from build123d import *

# Parameters (mm, degrees)
F0_R     = 3
F1_DEPTH = 2
F2_DEPTH = 5
F3_DEPTH = 9
F4_R     = 2.5
F5_DEPTH = 4
F7_DEPTH = 1
F10_D    = 2


with BuildPart() as f1:
    # F0 (on Front) → F1 (new body)
    with BuildSketch(Plane.XZ):
        with BuildLine():
            ThreePointArc((-5.5, 0), (0, 5.5), (5.5, 0))
            Line((5.5, 0), (5.5, 30))
            ThreePointArc((5.5, 30), (0, 35.5), (-5.5, 30))
            Line((-5.5, 30), (-5.5, 0))
        make_face()
        with Locations((0, 30)):
            Circle(F0_R, mode=Mode.SUBTRACT)
    extrude(amount=F1_DEPTH)

    # F0 (on Front) → F2 (join)
    with BuildSketch(Plane.XZ):
        with BuildLine():
            ThreePointArc((-5.5, 0), (0, -5.5), (5.5, 0))
            ThreePointArc((5.5, 0), (0, 5.5), (-5.5, 0))
        make_face()
        Polygon((2.8867513459, 0), (1.443375673, -2.5), (-1.443375673, -2.5), (-2.8867513459, 0), (-1.443375673, 2.5), (1.443375673, 2.5), align=None, mode=Mode.SUBTRACT)
    extrude(amount=F2_DEPTH)

    # F0 (on Front) → F3 (join)
    with BuildSketch(Plane.XZ):
        Polygon((-1.443375673, -2.5), (1.443375673, -2.5), (2.8867513459, 0), (1.443375673, 2.5), (-1.443375673, 2.5), (-2.8867513459, 0), align=None)
    extrude(amount=F3_DEPTH)

    # F4 (on face) → F5 (cut)
    with BuildSketch(Plane.XZ):
        Circle(F4_R)
    extrude(amount=F5_DEPTH, mode=Mode.SUBTRACT)

    # F6 (on Right) → F7 (join, symmetric)
    with BuildSketch(Plane.YZ):
        Polygon((-5, 5.5), (-5, 3.9388309233), (0, 3.9388309233), (0, 23.931786418), (-1.7340160995, 24.0223151183), align=None)
    extrude(amount=F7_DEPTH, both=True)

    # F10 (through all)
    with Locations(Plane(origin=(4.7631397208, 0, -2.75), x_dir=(0, 1, 0), z_dir=(0.8660254038, 0, -0.5))):
        with Locations((-2, 0)):
            Hole(F10_D / 2)


solid = f1.part
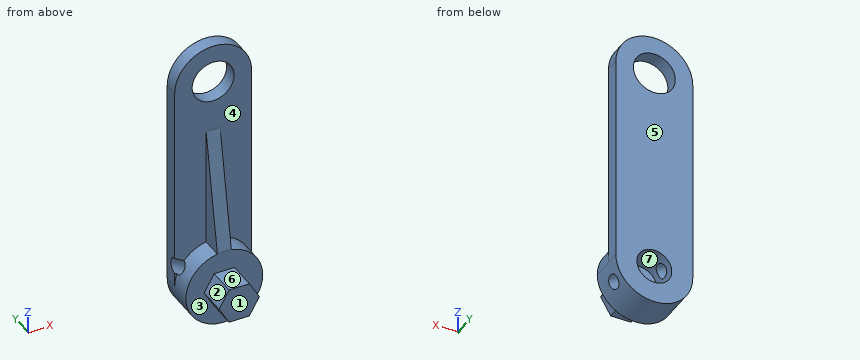
Here's how the part is built. I have some questions about the finished solid (model axes, mm). Face numbers are marked on the shaded views. A direction names the side the tool comes from. Coordinates: 2 decimals unless noted, no trailing zeros. Write each loop counter-clockwise with the first axis right and the second up, starting at its lowest first coordinate (ties: lowest second). Pieces come first, ordered by that corner, then holes.
1) If we section it at A-A (x = 0): List the corners of the cut face in (y, z) for me.
Filled in:
outline: (-9, -2.5) - (-5, -2.5) - (-5, -5.5) - (0, -5.5) - (0, -2.5) - (-4, -2.5) - (-4, 2.5) - (0, 2.5) - (0, 27) - (-2, 27) - (-2, 22.51) - (-5, 5.5) - (-5, 2.5) - (-9, 2.5) - close; (-2, 33) - (0, 33) - (0, 35.5) - (-2, 35.5) - close
2) If I drill on line 1 (Z direction, x = 0, y = -0.8); line 2 (Y direction, x = 3, z = 3.5); line 3 (Y direction, x = -2.5, z = 32.5), over which ranges is the centre line in solid material (lowest first)?
Filled in:
line 1: z = -5.5 to -2.5, 2.5 to 27, 33 to 35.5
line 2: y = -5 to 0
line 3: y = -2 to 0
3) I'm going to push flat-ended pins straight in: pin 1 (1.4 mm diameter, centred on x = 0, y = -6.5, fed in from +Z); pin 2 (5 mm diameter, centred on x = -4, y = -5.5, fed in from +Z); pin 3 (2.5 mm diameter, centred on x = -1, z = 0.5, fed in from +Y). Where does each tip first touch, or does it pass through?
Filled in:
pin 1: stops at z = 2.5
pin 2: stops at z = 5.28
pin 3: stops at y = -4
4) Which directions (+Z, -Z, +X, -X, +Y, -Y) give clear straight access to the entire face, cutting with the end or side of a thin tool? Please do the marked faces 1, 2, 3 and 4.
Filled in:
face 1: +Z, -Z, +X, -X, -Y
face 2: +Z, -X, -Y
face 3: -Y
face 4: +Z, -Y
5) If we section it at C-C (z = 11.5): List the corners of the cut face in (x, y) for me.
Filled in:
outline: (-5.5, -2) - (-1, -2) - (-1, -3.94) - (1, -3.94) - (1, -2) - (5.5, -2) - (5.5, 0) - (-5.5, 0) - close
6) Thinking about a two-plate mould opening in Z: for the marked faces 5, 6 and 7, which applies, +Z half, -Z half, draft (parallel to the pull), parting line (faces both ways), or undercut?
Filled in:
face 5: draft
face 6: +Z half
face 7: undercut
7) If we section it at B-B (y = -8): List the corners of the cut face in (x, z) for me, plus the area to 3 significant figures.
Filled in:
outline: (-2.89, 0) - (-1.44, -2.5) - (1.44, -2.5) - (2.89, 0) - (1.44, 2.5) - (-1.44, 2.5) - close
area: 21.7 mm2
